from build123d import *

# Parameters (mm, degrees)
F0_R     = 35
F1_DEPTH = 230
F3_R     = 40.5
F3_R_2   = 30.5
F4_DEPTH = 3
F6_R     = 40
F6_R_2   = 30.5
F7_DEPTH = 4
F8_R     = 40
F8_R_2   = 15
F9_DEPTH = 28


# Not quite as in the source:
# - a fillet or chamfer that OpenCascade refuses, or shapes differently, is made with other operations: its cross-section is extruded or revolved along the edge and cut away or added


with BuildPart() as f1:
    # F0 (on Front) → F1 (new body)
    with BuildSketch(Plane.XZ):
        Circle(F0_R)
    extrude(amount=-F1_DEPTH)

    # F3 (on offset) → F4 (cut)
    with BuildSketch(Plane.XZ.offset(-10)):
        Circle(F3_R)
        Circle(F3_R_2, mode=Mode.SUBTRACT)
    extrude(amount=-F4_DEPTH, mode=Mode.SUBTRACT)

    # F6 (on offset) → F7 (cut)
    with BuildSketch(Plane.XZ.offset(-94)):
        Circle(F6_R)
        Circle(F6_R_2, mode=Mode.SUBTRACT)
    extrude(amount=-F7_DEPTH, mode=Mode.SUBTRACT)

    # F8 (on face) → F9 (cut)
    with BuildSketch(Plane(origin=(0, 230, 0), x_dir=(-1, 0, 0), z_dir=(0, 1, 0))):
        Circle(F8_R)
        Circle(F8_R_2, mode=Mode.SUBTRACT)
    extrude(amount=-F9_DEPTH, mode=Mode.SUBTRACT)

    # F10: fillet of radius 30 on 1 edges, made by hand

    # F10_s1 → F10_t2 (revolve, cut)
    with BuildSketch(Plane.XY):
        with BuildLine():
            ThreePointArc((35, 173.7157287525), (29.4948974278, 191.0362368282), (15, 202))
            Line((15, 202), (35, 202))
            Line((35, 202), (35, 173.7157287525))
        make_face()
    revolve(axis=Axis((0, 202, 0), (0, -1, 0)), mode=Mode.SUBTRACT)


solid = f1.part
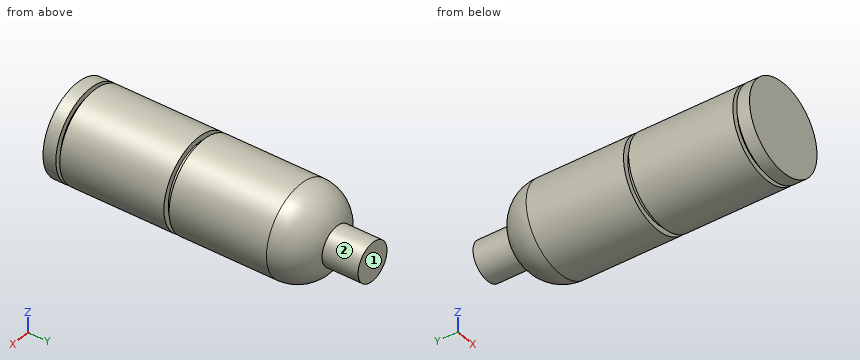
Work out the finished part from the listing and answer in its coordinate system (mm). Face numbers are marked on the shaded views. A direction names the side the tool comes from. Round coordinates to 2 decimals unless told otherwise and drop trailing zeros. Write each loop counter-clockwise with the first axis right and the second up, starting at its lowest first coordinate (ties: lowest second). Pieces come first, ordered by that corner, then holes. Notation, with made-up numbers: (16.5, 55.5) -> (31.5, 55.5) arc R13 cw to (31.5, 77.5) -> close; hole circle Ø8 at (-32, 11.5). An arc over 180 degrees is marked (long way). Write each question's results on one line, items separated by ' | '.
Item 1: Flat-ended cylindrical pins translate along their axes: P1, Ø1, axis at x = -1.5, y = 26.5, coming from the -Z side; P2, Ø8, axis at x = 20.5, y = 126, coming from the -Z side; P3, Ø6, axis at y = 192, z = -12, coming from the -X side. Find the tip coordinate at first contact, or state that the pin passes through.
Result set:
P1: z = -34.99 | P2: z = -30.87 | P3: x = -28.71
Item 2: A cutting plane is placed at A-A, the plane y = 161.5. Determine the outline of the cut face in (x, z).
Result set:
outline: circle Ø70 at (0, 0)
Item 3: Find the intervals of material crossed by line 1 along Z through (x, y) = (1.5, 51); line 2 along Y through (x, z) = (18.5, 27); line 3 along Z through (x, y) = (-25, 11), in increasing order. Write a range as [from, to].
Result set:
line 1: [-34.97, 34.97] | line 2: [0, 10], [13, 94], [98, 185.16] | line 3: [-17.47, 17.47]
Item 4: Which of the six approach directions +Z, -Z, +X, -X, +Y, -Y give full straight-line access (tool end or side, diameter ignored) to the marked faces 1 and 2?
Result set:
face 1: +Z, -Z, +X, -X, +Y | face 2: +Y
